Autodesk Inventor part; units mm, degrees
ref_plane "YZ Plane" through (0, 0, 0) normal (1, 0, 0) x (0, 1, 0)
ref_plane "XZ Plane" through (0, 0, 0) normal (0, 1, 0) x (-1, 0, 0)
ref_plane "XY Plane" through (0, 0, 0) normal (0, 0, 1) x (1, 0, 0)
sketch "Sketch1" plane through (0, 0, 0) normal (0, 1, 0) x (-1, 0, 0)
  circle A0 centre (0, 0) radius 26
  circle A1 centre (0, 0) radius 31
  dimension "d0" = 52
  dimension "d1" = 62
extrude "Extrusion1" add sketch "Sketch1" along normal blind 27
sketch "Sketch2" plane through (0, 27, 0) normal (0, 1, 0) x (1, 0, 0)
  circle A0 centre (0, 0) radius 25
  circle A1 centre (0, 0) radius 31
  dimension "d4" = 50
extrude "Extrusion2" add sketch "Sketch2" along normal blind 5
sketch "Sketch3" plane through (0, 32, 0) normal (0, 1, 0) x (1, 0, 0)
  circle A0 centre (0, 0) radius 31
  circle A1 centre (0, 0) radius 26
extrude "Extrusion3" add sketch "Sketch3" along normal blind 7
properties part number "Axis 4 Female Bearing Connector Bracket"
Check sheet for the modelled part. Datum: model origin and axes. Units: mm. A direction names the side the tool comes from. Give positions to 0.01 mm unless a question says otherwise; leave off trailing zeros. Order: outer loops, then holes, each group sorted by start corner. A loop starts at its lowest first (then second) coordinate and runs counter-clockwise, first axis right, second up. Notation, with made-up numbers: M 15.25,28 L 74.25,28 A30 cw 74.25,60 Z; hole C 88.25,-19 d4. An arc over 180 degrees is marked long. Answer in a Markdown table with one row per item. Add a question column.
Q1. Access from +Z, -Z, +X, -X, +Y, -Y to the whole of each face (thin tool, end or side, straight path). Record for faces 3 (the flat face through (-14, 27, -21)), 4 (the cylindrical face through (-20.633, 35.451, -15.821)), 5 (the cylindrical face through (23.846, 29.465, 7.509)).
Q2. Release check for a two-part mould opening along Z. For faces 1 (the cylindrical face through (20.633, 13.311, 15.821)), 2 (the flat face through (-16, 39, 21)) record: released by +Z, released by -Z, zero draft, split by the parting line, or undercut.
Q3. Sectioned sample at D-D, the plane z = -12.5. Record the boundary of the cut face in (x, y).
Q4. Gauge pin test, flat ends, axial feed: pin 1 Ø1.5 at (y, z) = (17, -3) entering from -X; pin 2 Ø4 at (x, y) = (-11, 18) entering from -Z; pin 3 Ø1 at (y, z) = (15.5, -4.5) entering from -X. Record the tip position at first contact, or that the pin passes through.
Q5. Thickness scan on L1, parallel to Z at x = 0, y = 21.25; L2, parallel to X at y = 28, z = 0. Record the ranges inside material, lowest first.
Q6. Sectioned sample at B-B, the plane y = 8. Record the boundary of the cut face in (x, z), and give its area (3 significant figures).
Q7. Sectioned sample at A-A, the plane z = -22.5. Record the boundary of the cut face in (x, y).
Verdict:
| question | item | result |
|---|---|---|
| 1 | face 3 | -Y |
| 1 | face 4 | +Y |
| 1 | face 5 | +Y, -Y |
| 2 | face 1 | undercut |
| 2 | face 2 | zero draft |
| 3 | outline | M -28.37,0 L -22.8,0 L -22.8,27 L -21.65,27 L -21.65,32 L -22.8,32 L -22.8,39 L -28.37,39 Z; M 21.65,27 L 22.8,27 L 22.8,0 L 28.37,0 L 28.37,39 L 22.8,39 L 22.8,32 L 21.65,32 Z |
| 4 | pin 1 | x = -30.92 |
| 4 | pin 2 | z = -29.66 |
| 4 | pin 3 | x = -30.74 |
| 5 | L1 | -31 to -26, 26 to 31 |
| 5 | L2 | -31 to -25, 25 to 31 |
| 6 | outline | C 0,0 d62; hole C 0,0 d52 |
| 6 | area | 895 mm² |
| 7 | outline | M -21.32,0 L -13.03,0 L -13.03,27 L -10.9,27 L -10.9,32 L -13.03,32 L -13.03,39 L -21.32,39 Z; M 10.9,27 L 13.03,27 L 13.03,0 L 21.32,0 L 21.32,39 L 13.03,39 L 13.03,32 L 10.9,32 Z |
